Design review of the part built by this model. Coordinates are the model's own, in mm. Face numbers are marked on the shaded views. Give positions to 0.01 mm unless a question says otherwise; leave off trailing zeros. Write each loop counter-clockwise with the first axis right and the second up, starting at its lowest first coordinate (ties: lowest second). Pieces come first, ordered by that corner, then holes. Notation, with made-up numbers: M 87,48.5 L 107,48.5 A30 cw 107,77.5 Z; hole C 29,-8 d4. An arc over 180 degrees is marked long. Use one line per item in the form item = value. Start each with the question number.
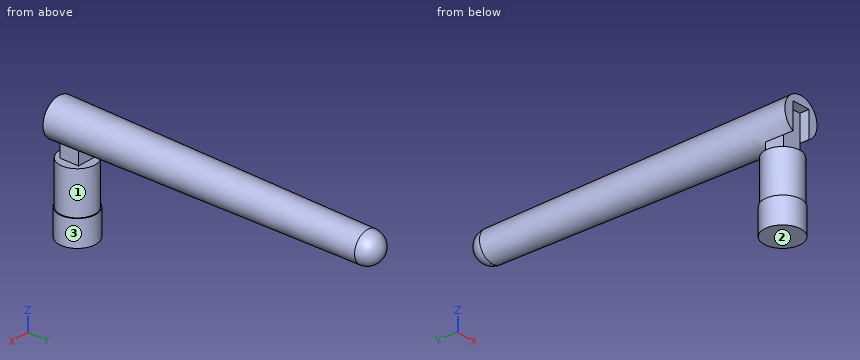
from build123d import *

# Parameters (mm, degrees)
SKETCH1_R           = 5
BOSS_EXTRUDE1_DEPTH = 7
SKETCH2_R           = 4.75
BOSS_EXTRUDE2_DEPTH = 11.5
SKETCH5_W           = 5
SKETCH5_H           = 5
BOSS_EXTRUDE3_DEPTH = 10.5
SKETCH6_W           = 5
SKETCH6_H           = 10.5
CUT_EXTRUDE1_DEPTH  = 2.5


with BuildPart() as part:
    # Sketch1 → Boss-Extrude1 (new body)
    with BuildSketch(Plane.XY):
        Circle(SKETCH1_R)
    extrude(amount=BOSS_EXTRUDE1_DEPTH)

    # Sketch2 → Boss-Extrude2 (add)
    with BuildSketch(Plane.XY.offset(7)):
        Circle(SKETCH2_R)
    extrude(amount=BOSS_EXTRUDE2_DEPTH)



with BuildPart() as body_2:
    # Sketch4 → Revolve2 (revolve)
    with BuildSketch(Plane.XY.offset(26.25), mode=Mode.PRIVATE) as revolve2_sk:
        with BuildLine():
            Line((0, -5), (-5, -5))
            Line((-5, -5), (-4.045451611, 79.000258239))
            ThreePointArc((-4.045451611, 79.000258239), (-2.844451304, 81.831245462), (0, 83))
            Line((0, 83), (0, -5))
        make_face()
    revolve(revolve2_sk.sketch.rotate(Axis((0, -1000, 26.25), (0, 1, 0)), 180), axis=Axis((0, -1000, 26.25), (0, 1, 0)))


with BuildPart() as part_1:
    add(part.part)

    add(body_2.part)  # Boss-Extrude3 merges body 2
    # Sketch5 → Boss-Extrude3 (add)
    with BuildSketch(Plane.XY.offset(18.5)):
        Rectangle(SKETCH5_W, SKETCH5_H)
    extrude(amount=BOSS_EXTRUDE3_DEPTH)

    # Sketch6 → Cut-Extrude1 (cut)
    with BuildSketch(Plane.XZ.offset(5)):
        with Locations((0, 23.75)):
            Rectangle(SKETCH6_W, SKETCH6_H)
    extrude(amount=-CUT_EXTRUDE1_DEPTH, mode=Mode.SUBTRACT)


solid = part_1.part
1. To check wall thickness, follow L1, parallel to Y at x = -1, z = 20.5; L2, parallel to Y at x = 0, z = 2.5; L3, parallel to Z at x = 4, y = 46. State the ranges of each line that lie inside material, in increasing order.
2. We need section A-A (y = 0). State the section outline as (x, z) points.
3. Clearance check with flat-ended pins moving along their axes: pin 1 Ø4 at (y, z) = (47.5, 25) entering from -X; pin 2 Ø3 at (x, z) = (-3.5, 16.5) entering from +Y; pin 3 Ø2 at (x, y) = (4, 72.5) entering from -Z. State where each tip first meets the part, or that it passes through.
4. We need section B-B (z = 6). State the section outline as (x, y) points.
5. Draft analysis for pull direction Z (two halves, no side actions). For the marked faces 1, 2 and 3, state which applies: pulls with the +Z half, pulls with the -Z half, needs draft (parallel to the pull), parting line crosses it, or undercut.
6. We need section C-C (z = 11). State the section outline as (x, y) points, and give its area (3 significant figures).
Answer block:
q1.L1 = -2.5 to 2.5
q1.L2 = -5 to 5
q1.L3 = 24.37 to 28.13
q2.outline = M -5,0 L 5,0 L 5,7 L 4.75,7 L 4.75,18.5 L 2.5,18.5 L 2.5,21.99 A4.94 ccw long -2.5,21.99 L -2.5,18.5 L -4.75,18.5 L -4.75,7 L -5,7 Z
q3.pin_1 = -4.42
q3.pin_2 = 4.31
q3.pin_3 = 23.43
q4.outline = C 0,0 d10
q5.face_1 = undercut
q5.face_2 = pulls with the -Z half
q5.face_3 = needs draft
q6.outline = C 0,0 d9.5
q6.area = 70.9 mm^2
